```python
from build123d import *

# Parameters (mm, degrees)
SKETCH1_W           = 55
SKETCH1_H           = 25
SKETCH1_R           = 3.5
BOSS_EXTRUDE1_DEPTH = 2
SKETCH2_W           = 25
SKETCH2_H           = 51.88
SKETCH2_R           = 3.5
BOSS_EXTRUDE2_DEPTH = 2
FILLET2_R           = 40
SKETCH5_W           = 13
SKETCH5_H           = 25
SKETCH5_R           = 3.5
BOSS_EXTRUDE5_DEPTH = 17.7
SKETCH6_W           = 25
SKETCH6_H           = 9.88
SKETCH6_R           = 3.5
BOSS_EXTRUDE6_DEPTH = 17.7
FILLET3_R           = 2
FILLET4_R           = 2


with BuildPart() as part:
    # Sketch1 → Boss-Extrude1 (new body)
    with BuildSketch(Plane(origin=(0, 0, 0), x_dir=(1, 0, 0), z_dir=(0, 1, 0))):
        with Locations((22.5, 3)):
            Rectangle(SKETCH1_W, SKETCH1_H)
        with Locations(Location((0, 0, 0), (0, 0, 270))):
            Circle(SKETCH1_R, mode=Mode.SUBTRACT)
    extrude(amount=BOSS_EXTRUDE1_DEPTH)

    # Sketch2 → Boss-Extrude2 (add)
    with BuildSketch(Plane(origin=(50, 0, 0), x_dir=(0, 0, -1), z_dir=(1, 0, 0))):
        with Locations((3, 25.94)):
            Rectangle(SKETCH2_W, SKETCH2_H)
        with Locations((0, 46.88)):
            Circle(SKETCH2_R, mode=Mode.SUBTRACT)
    extrude(amount=-BOSS_EXTRUDE2_DEPTH)

    # Fillet2
    fillet2_edges = [part.edges().sort_by_distance(p)[0] for p in [
        (48, 2, -3),
        (50, 0, -3),
    ]]
    fillet(fillet2_edges, radius=FILLET2_R)

    # Sketch5 → Boss-Extrude5 (add)
    with BuildSketch(Plane(origin=(0, 2, 0), x_dir=(1, 0, 0), z_dir=(0, 1, 0))):
        with Locations((1.5, 3)):
            Rectangle(SKETCH5_W, SKETCH5_H)
        with Locations(Location((0, 0, 0), (0, 0, 270))):
            Circle(SKETCH5_R, mode=Mode.SUBTRACT)
    extrude(amount=BOSS_EXTRUDE5_DEPTH)

    # Sketch6 → Boss-Extrude6 (add)
    with BuildSketch(Plane.ZY.offset(-48)):
        with Locations((-3, 46.94)):
            Rectangle(SKETCH6_W, SKETCH6_H)
        with Locations(Location((0, 46.88, 0), (0, 0, 180))):
            Circle(SKETCH6_R, mode=Mode.SUBTRACT)
    extrude(amount=BOSS_EXTRUDE6_DEPTH)

    # Fillet3
    fillet3_edges = [part.edges().sort_by_distance(p)[0] for p in [
        (48, 42, -3),
    ]]
    fillet(fillet3_edges, radius=FILLET3_R)

    # Fillet4
    fillet4_edges = [part.edges().sort_by_distance(p)[0] for p in [
        (8, 2, -3),
    ]]
    fillet(fillet4_edges, radius=FILLET4_R)


solid = part.part
```
CAD build for the part. Positions are in the model's coordinates, mm. A direction names the side the tool comes from. Give positions to 0.01 mm unless a question says otherwise; leave off trailing zeros. Order: outer loops, then holes, each group sorted by start corner. A loop starts at its lowest first (then second) coordinate and runs counter-clockwise, first axis right, second up. Notation, with made-up numbers: M 69,55.5 L 82,55.5 A29 cw 82,76.5 Z; hole C -18.5,53.5 d5. An arc over 180 degrees is marked long. Put each result on its own line as item: value. Start each with the question number.
(1) Saw through at A-A, the plane x = 0. Write the cut outline in (y, z), then the cut area to 3 significant figures.
(2) Which spindle directions (+Z, -Z, +X, -X, +Y, -Y) get a long thin tool onto all of the face, cutting with end or side? Do faces 5 (the flat face through (2.4, 0, -3.2)), 6 (the flat face through (30.3, 47, -6)), 7 (the flat face through (38, 42, -3)). Say none if no direction does.
(3) Drill centre lines: line 1 along X through (y, z) = (6, 0); line 2 along Z through (x, y) = (37, 46.88); line 3 along Y through (x, z) = (43, -1). Where is each one in solid material? Low to high.
(4) Saw through at D-D, the plane y = 46.88. Write the cut outline in (x, z).
(5) Saw through at C-C, the plane z = 0. Write the cut outline in (x, y), then the cut area to 3 significant figures.
(6) Saw through at B-B, the plane y = 16. Write the cut outline in (x, z).
(7) Flat gauge pins, fed straight in: pin 1 Ø12.5 at (y, z) = (8, -3.5) entering from +X; pin 2 Ø4.5 at (x, z) = (37, -8) entering from -Y; pin 3 Ø12 at (y, z) = (35.5, -12.5) entering from -X. Where does each tip first touch, or does it go through?
(8) Mould opens along Y. For faces 1 (the cylindrical face through (47.414, 41.36, -3.175)), 2 (the flat face through (8, 12, -3)), 3 (the cylindrical face through (8.64, 2.586, -3.175)), 4 (the cylindrical face through (36.573, 14.007, -3.175)) say: +Y half, -Y half, draft (parallel to the pull), parting line (faces both ways), or undercut.
Check result:
1. outline: M 0,-15.5 L 19.7,-15.5 L 19.7,-3.5 L 0,-3.5 Z; M 0,3.5 L 19.7,3.5 L 19.7,9.5 L 0,9.5 Z
1. area: 355 mm2
2. face 5: +Z, -Z, +X, -X, -Y
2. face 6: +Z, -Z, -X, +Y
2. face 7: +Z, -Z, -X
3. line 1: x = -5 to -3.5, 3.5 to 8, 25.44 to 31.07
3. line 2: z = -15.5 to -3.5, 3.5 to 9.5
3. line 3: y = 17.39 to 22.64, 42 to 43.53, 50.23 to 51.88
4. outline: M 30.3,-15.5 L 50,-15.5 L 50,-3.5 L 30.3,-3.5 Z; M 30.3,3.5 L 50,3.5 L 50,9.5 L 30.3,9.5 Z
5. outline: M -5,0 L -3.5,0 L -3.5,19.7 L -5,19.7 Z; M 3.5,0 L 10,0 A40 ccw 50,40 L 50,43.38 L 30.3,43.38 L 30.3,42 L 45.95,42 A2 cw 47.94,39.89 A40 cw 10.11,2.06 A2 cw 8,4.05 L 8,19.7 L 3.5,19.7 Z; M 30.3,50.38 L 50,50.38 L 50,51.88 L 30.3,51.88 Z
5. area: 341 mm2
6. outline: M -5,-15.5 L 8,-15.5 L 8,9.5 L -5,9.5 Z; M 38.4,-15.5 L 42,-15.5 L 42,9.5 L 38.4,9.5 Z; hole C 0,0 d7
7. pin 1: stops at x = 40.61
7. pin 2: stops at y = 8.58
7. pin 3: stops at x = 46
8. face 1: undercut
8. face 2: draft
8. face 3: +Y half
8. face 4: undercut
